from build123d import *

# Parameters (mm, degrees)
SKETCH1_R                = 110
SKETCH1_R_2              = 6.35
BOSS_EXTRUDE1_DEPTH      = 1.5875
CUT_EXTRUDE3_DEPTH       = 156.595888844
CIRPATTERN1_COUNT        = 2
CIRPATTERN2_COUNT        = 2
CIRPATTERN2_ANGLE        = 60
CIRPATTERN2_COPY_1_DEPTH = 156.595888844
CUT_EXTRUDE5_DEPTH       = 155.188458145


with BuildPart() as part:
    # Sketch1 → Boss-Extrude1 (new, symmetric)
    with BuildSketch(Plane.XY):
        Circle(SKETCH1_R)
        Circle(SKETCH1_R_2, mode=Mode.SUBTRACT)
        Polygon((-6.35, 40), (-3.85, 40), (-3.85, 48), (-0.85, 48), (-0.85, 93), (-20.85, 93), (-20.85, 40), (-18.35, 40), align=None, mode=Mode.SUBTRACT)
        Polygon((6.35, -40), (3.85, -40), (3.85, -48), (0.85, -48), (0.85, -93), (20.85, -93), (20.85, -40), (18.35, -40), align=None, mode=Mode.SUBTRACT)
        Polygon((37.816016151, -14.500738686), (36.566016151, -16.665802195), (43.494219382, -20.665802195), (41.994219382, -23.263878407), (80.965362552, -45.763878407), (90.965362552, -28.443370331), (45.066016151, -1.943370331), (43.816016151, -4.108433841), align=None, mode=Mode.SUBTRACT)
        Polygon((-37.816016151, 14.500738686), (-36.566016151, 16.665802195), (-43.494219382, 20.665802195), (-41.994219382, 23.263878407), (-80.965362552, 45.763878407), (-90.965362552, 28.443370331), (-45.066016151, 1.943370331), (-43.816016151, 4.108433841), align=None, mode=Mode.SUBTRACT)
    extrude(amount=BOSS_EXTRUDE1_DEPTH, both=True)

    # Sketch2 → Cut-Extrude3 (cut, through all)
    with BuildSketch(Plane.XY.offset(1.5875)):
        with BuildLine():
            Line((-50.613025421, -97.664331553), (-37.85, -75.558123066))
            Line((-37.85, -75.558123066), (-9.15, -75.558123066))
            Line((-9.15, -75.558123066), (-9.15, -103))
            Line((-9.15, -103), (5.85, -103))
            ThreePointArc((5.85, -103), (10.85, -108), (15.85, -103))
            Line((15.85, -103), (30.85, -103))
            Line((30.85, -103), (30.85, -75.558123066))
            Line((30.85, -75.558123066), (37.85, -75.558123066))
            Line((37.85, -75.558123066), (50.613025421, -97.664331553))
            ThreePointArc((50.613025421, -97.664331553), (0, -110), (-50.613025421, -97.664331553))
        make_face()
    cut_extrude3 = extrude(amount=-CUT_EXTRUDE3_DEPTH, mode=Mode.SUBTRACT)

    # CirPattern1: Cut-Extrude3 ×2 about axis
    cirpattern1_axis = Axis((0, 0, 0), (0, 0, 1))
    for i in range(1, CIRPATTERN1_COUNT):
        add(cut_extrude3.rotate(cirpattern1_axis, i * 360 / CIRPATTERN1_COUNT), mode=Mode.SUBTRACT)

    # CirPattern2: Cut-Extrude3 ×2 about axis
    cirpattern2_axis = Axis((0, 0, 0), (0, 0, 1))
    for i in range(1, CIRPATTERN2_COUNT):
        add(cut_extrude3.rotate(cirpattern2_axis, i * CIRPATTERN2_ANGLE / (CIRPATTERN2_COUNT - 1)), mode=Mode.SUBTRACT)

    # CirPattern2 copy 1 sketch → CirPattern2 copy 1 (cut, through all)
    with BuildSketch(Plane(origin=(0, 0, 1.5875), x_dir=(-0.4999999999999979, -0.8660254037844398, 0), z_dir=(0, 0, 1))):
        with BuildLine():
            Line((-50.613025421, -97.664331553), (-37.85, -75.558123066))
            Line((-37.85, -75.558123066), (-9.15, -75.558123066))
            Line((-9.15, -75.558123066), (-9.15, -103))
            Line((-9.15, -103), (5.85, -103))
            ThreePointArc((5.85, -103), (10.85, -108), (15.85, -103))
            Line((15.85, -103), (30.85, -103))
            Line((30.85, -103), (30.85, -75.558123066))
            Line((30.85, -75.558123066), (37.85, -75.558123066))
            Line((37.85, -75.558123066), (50.613025421, -97.664331553))
            ThreePointArc((50.613025421, -97.664331553), (0, -110), (-50.613025421, -97.664331553))
        make_face()
    extrude(amount=-CIRPATTERN2_COPY_1_DEPTH, mode=Mode.SUBTRACT)

    # Sketch5 → Cut-Extrude5 (cut, through all)
    with BuildSketch(Plane.XY.offset(1.5875)):
        with BuildLine():
            Line((-109.544511501, -10), (-84.014511501, -10))
            Line((-84.014511501, -10), (-50.667509788, -67.758701246))
            Line((-50.667509788, -67.758701246), (-63.432509788, -89.868329805))
            ThreePointArc((-63.432509788, -89.868329805), (-95.262794416, -55), (-109.544511501, -10))
        make_face()
        with BuildLine():
            Line((109.544511501, 10), (84.014511501, 10))
            Line((84.014511501, 10), (50.667509788, 67.758701246))
            Line((50.667509788, 67.758701246), (63.432509788, 89.868329805))
            ThreePointArc((63.432509788, 89.868329805), (95.262794416, 55), (109.544511501, 10))
        make_face()
    extrude(amount=-CUT_EXTRUDE5_DEPTH, mode=Mode.SUBTRACT)


solid = part.part
Work out the finished part from the listing and answer in its coordinate system (mm). A direction names the side the tool comes from. Coordinates: 2 decimals unless noted, no trailing zeros. Loops run counter-clockwise (first coordinate to the right, second up) from the corner with the lowest first, then second, coordinate; pieces in that order, holes last. Notation, with made-up numbers: M -29,-12.75 L -4,-12.75 A14 cw -4,14.25 Z; hole C 17.25,8.25 d2. An arc over 180 degrees is marked long. Answer in a Markdown table with one row per item. Add a question column.
1. The mould has two halves that part along Y. Classify faces 5 (the cylindrical face through (-57.25, -93.93, 0.02)), 6 (the flat face through (-2, -22, -1.588)), 7 (the flat face through (68.34, -15.38, 0.02)), 8 (the flat face through (-44.142, 86.456, 0.022)): pulls with the +Y half, pulls with the -Y half, needs draft (parallel to the pull), parting line crosses it, or undercut.
2. Flat-ended cylindrical pins translate along their axes: P1, Ø1.6, axis at y = 55, z = 0, coming from the +X side; P2, Ø1.6, axis at x = -35, z = -0.5, coming from the +Y side; P3, Ø1, axis at y = 43.5, z = 0.5, coming from the -X side. Find the tip coordinate at first contact, or state that the pin passes through.
3. Find section B-B, the plane y = 85.5. Write down the section's boundary in (x, z).
4. Find section A-A, the plane y = -42.5. Write down the section's boundary in (x, z).
5. Consider L1, parallel to Y at x = 16, z = -0.2; L2, parallel to X at y = 58, z = -0.5; L3, parallel to Y at x = 0, z = -0.3. Determine where each line is inside the solid, lowest interval first.
6. Find section C-C, the plane z = -1. State how many separate pieces and enclosed holes the cut face has, then the cut area to 3 significant figures.
7. A tool of negligible diameter and unlimited length cuts with its end or side. For faces 1 (the flat face through (85.9, -37.22, 0.02)), 2 (the flat face through (53, -81.8, 0)), 3 (the flat face through (-56.96, -78.66, 0.02)), 4 (the flat face through (72.58, -52.47, 0.02)), from which of +Z, -Z, +X, -X, +Y, -Y can it reach the whole face along a straight path? Write none if from no direction.
Reported:
| question | item | result |
|---|---|---|
| 1 | face 5 | pulls with the -Y half |
| 1 | face 6 | needs draft |
| 1 | face 7 | undercut |
| 1 | face 8 | pulls with the +Y half |
| 2 | P1 | stops at x = 58.5 |
| 2 | P2 | stops at y = 75.56 |
| 2 | P3 | stops at x = -99.54 |
| 3 | outline | M -55.14,-1.59 L -43.59,-1.59 L -43.59,1.59 L -55.14,1.59 Z; M -30.85,-1.59 L -20.85,-1.59 L -20.85,1.59 L -30.85,1.59 Z; M -0.85,-1.59 L 9.15,-1.59 L 9.15,1.59 L -0.85,1.59 Z; M 43.59,-1.59 L 60.91,-1.59 L 60.91,1.59 L 43.59,1.59 Z |
| 4 | outline | M -65.25,-1.59 L 3.85,-1.59 L 3.85,1.59 L -65.25,1.59 Z; M 20.85,-1.59 L 75.31,-1.59 L 75.31,1.59 L 20.85,1.59 Z; M 82.85,-1.59 L 99.61,-1.59 L 99.61,1.59 L 82.85,1.59 Z |
| 5 | L1 | y = -103 to -93, -40 to 75.56 |
| 5 | L2 | x = -85.45 to -82.16, -53.76 to -20.85, -0.85 to 56.3 |
| 5 | L3 | y = -103 to -6.35, 6.35 to 103 |
| 6 | separate pieces | 1 |
| 6 | enclosed holes | 5 |
| 6 | area | 22,300 mm^2 |
| 7 | face 1 | +Z, -Z |
| 7 | face 2 | +Z, -Z, +X |
| 7 | face 3 | +Z, -Z, -X |
| 7 | face 4 | +Z, -Z, -Y |
